```python
from build123d import *

# Parameters (mm, degrees)
F2_R          = 8
F3_DEPTH      = 55
F5_DEPTH      = 6
F7_DEPTH      = 5
F7_DEPTH_BACK = 11


# Not quite as in the source:
# - a pattern or mirror of a feature is missing from the dataset's text; its kind, count and spacing are read off the source's solid


with BuildPart() as f1:
    # F0 (on Front) → F1 (revolve)
    with BuildSketch(Plane.XZ):
        with BuildLine():
            Line((0, -25), (0, 25))
            ThreePointArc((0, 25), (-25, 0), (0, -25))
        make_face()
    revolve(axis=Axis((0, 0, 0), (0, 0, -1)))

    # F2 (on Right) → F3 (join)
    with BuildSketch(Plane.YZ):
        Circle(F2_R)
    f3 = extrude(amount=F3_DEPTH)

    # F3_copies: F3 across plane
    add(f3.mirror(Plane(origin=(0, 0, 0), x_dir=(0, 0, -1), z_dir=(-1, 0, 0))))

    # F4 (on face) → F5 (join)
    with BuildSketch(Plane.YZ.offset(55)):
        Polygon((-42.1359225246, 90), (-70, 0), (-42.1359225246, -90), (42.1359225246, -90), (70, 0), (42.1359225246, 90), align=None)
    f5 = extrude(amount=F5_DEPTH)

    # F5_copies: F5 across plane
    add(f5.mirror(Plane(origin=(0, 0, 0), x_dir=(0, 0, -1), z_dir=(-1, 0, 0))))

    # F6 (on face) → F7 (join, two sides)
    with BuildSketch(Plane.YZ.offset(61)) as f7_sk:
        Polygon((-11.5470053838, -20), (11.5470053838, -20), (23.0940107676, 0), (11.5470053838, 20), (-11.5470053838, 20), (-23.0940107676, 0), align=None)
    f7 = extrude(amount=F7_DEPTH) + extrude(f7_sk.sketch, amount=-F7_DEPTH_BACK)

    # F7_copies: F7 across plane
    add(f7.mirror(Plane(origin=(0, 0, 0), x_dir=(0, 0, -1), z_dir=(-1, 0, 0))))


solid = f1.part
```
Could you check a few things on this model? Use its own coordinates, in mm. A direction names the side the tool comes from. Round coordinates to 2 decimals unless told otherwise and drop trailing zeros. Write each loop counter-clockwise with the first axis right and the second up, starting at its lowest first coordinate (ties: lowest second). Pieces come first, ordered by that corner, then holes. Notation, with made-up numbers: M 74,17 L 107,17 A20 cw 107,31 Z; hole C 64,67 d10. An arc over 180 degrees is marked long. Write each question's results on one line, items separated by ' | '. Start each with the question number.
1. I'm going to push flat-ended pins straight in: pin 1 Ø1.5 at (x, y) = (-53.5, -0.5) entering from -Z; pin 2 Ø2 at (x, y) = (-5, -6) entering from +Z; pin 3 Ø6 at (y, z) = (-2, 70.5) entering from +X. Where does each tip first touch, or does it pass through?
2. Imagine slicing it at C-C on y = 15. List the corners of the cut face in (x, z) for me.
3. On a 3-axis mill with a long thin cutter (end or side, diameter ignored), from which of +Z, -Z, +X, -X, +Y, -Y can I reach the whole of each face in a straight line? I mean faces 4 (the face through (-52, 0, 20)), 5 (the face through (-52.46, 17.24, -10.14)), 6 (the face through (53, 0, -20)). Say none if no direction works.
4. I need wall thicknesses on L1, parallel to X at y = 13.5, z = -70.5; L2, parallel to Z at x = -39, y = 6; L3, parallel to Y at x = 59, z = 25. Which ranges of each line are inside material? Lowest first, please. Write a range as from..to.
5. Imagine slicing it at D-D on z = 29. List the corners of the cut face in (x, y) for me.
6. Thinking about a two-plate mould opening in X: for faces 1 (the face through (-57.958, 55.873, -45.63)), 2 (the face through (66, 0, 0)), 3 (the face through (-50, 10, 0)), which applies, +X half, -X half, draft (parallel to the pull), parting line (faces both ways), or undercut?
7. Imagine slicing it at A-A on z = -69.5. List the corners of the cut face in (x, y) for me.
Result sheet:
1) pin 1: stops at z = -20 | pin 2: stops at z = 24.05 | pin 3: stops at x = 61
2) outline: M -66,-14.02 L -61,-14.02 L -61,-90 L -55,-90 L -55,-14.02 L -50,-14.02 L -50,14.02 L -55,14.02 L -55,90 L -61,90 L -61,14.02 L -66,14.02 Z; C 0,0 d40; M 50,-14.02 L 55,-14.02 L 55,-90 L 61,-90 L 61,-14.02 L 66,-14.02 L 66,14.02 L 61,14.02 L 61,90 L 55,90 L 55,14.02 L 50,14.02 Z
3) face 4: +Z, +Y, -Y | face 5: -Z, +Y | face 6: -Z, +Y, -Y
4) L1: x = -61..-55, 55..61 | L2: z = -5.29..5.29 | L3: y = -62.26..62.26
5) outline: M -61,-61.02 L -55,-61.02 L -55,61.02 L -61,61.02 Z; M 55,-61.02 L 61,-61.02 L 61,61.02 L 55,61.02 Z
6) face 1: draft | face 2: +X half | face 3: undercut
7) outline: M -61,-48.48 L -55,-48.48 L -55,48.48 L -61,48.48 Z; M 55,-48.48 L 61,-48.48 L 61,48.48 L 55,48.48 Z
